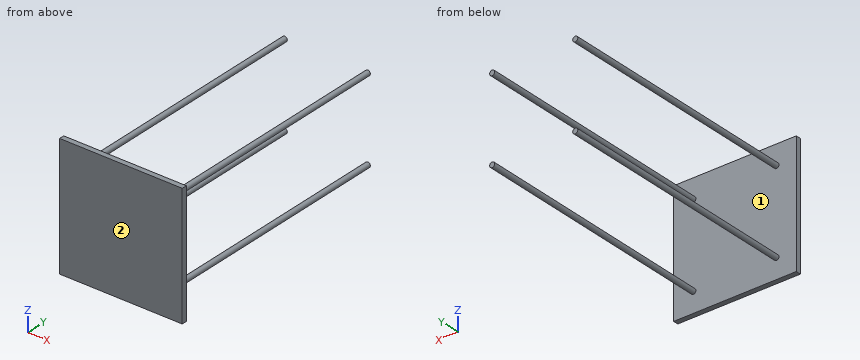
```python
from build123d import *

# Parameters (mm, degrees)
SKETCH1_W           = 120
SKETCH1_H           = 120
SKETCH1_R           = 2.5
BOSS_EXTRUDE1_DEPTH = 5
SKETCH1_3_R         = 2.5
BOSS_EXTRUDE2_DEPTH = 250


with BuildPart() as part:
    # Sketch1 → Boss-Extrude1 (new body)
    with BuildSketch(Plane(origin=(0, 0, 0), x_dir=(1, 0, 0), z_dir=(0, 1, 0))):
        Rectangle(SKETCH1_W, SKETCH1_H)
        with Locations(Location((-40.658639918, -40.658639918, 0), (0, 0, 270))):
            Circle(SKETCH1_R, mode=Mode.SUBTRACT)
        with Locations(Location((40.658639918, 40.658639918, 0), (0, 0, 270))):
            Circle(SKETCH1_R, mode=Mode.SUBTRACT)
        with Locations(Location((40.658639918, -40.658639918, 0), (0, 0, 270))):
            Circle(SKETCH1_R, mode=Mode.SUBTRACT)
        with Locations(Location((-40.658639918, 40.658639918, 0), (0, 0, 270))):
            Circle(SKETCH1_R, mode=Mode.SUBTRACT)
    extrude(amount=BOSS_EXTRUDE1_DEPTH)

    # Sketch1_3 → Boss-Extrude2 (add)
    with BuildSketch(Plane(origin=(0, 0, 0), x_dir=(1, 0, 0), z_dir=(0, 1, 0))):
        with Locations(Location((-40.658639918, -40.658639918, 0), (0, 0, 270))):
            Circle(SKETCH1_3_R)
        with Locations(Location((-40.658639918, 40.658639918, 0), (0, 0, 270))):
            Circle(SKETCH1_3_R)
        with Locations(Location((40.658639918, 40.658639918, 0), (0, 0, 270))):
            Circle(SKETCH1_3_R)
        with Locations(Location((40.658639918, -40.658639918, 0), (0, 0, 270))):
            Circle(SKETCH1_3_R)
    extrude(amount=BOSS_EXTRUDE2_DEPTH)


solid = part.part
```
For this review, take the finished solid that the model builds, in its own axes (mm). Face numbers are marked on the shaded views. A direction names the side the tool comes from. Round coordinates to 2 decimals unless told otherwise and drop trailing zeros. Write each loop counter-clockwise with the first axis right and the second up, starting at its lowest first coordinate (ties: lowest second). Pieces come first, ordered by that corner, then holes.
1) Take a section at B-B on z = 28.5. Give the boundary of the cut face in (x, y), then the cut area to 3 significant figures.
Answer below:
outline: (-60, 0) - (60, 0) - (60, 5) - (-60, 5) - close
area: 600 mm2
2) Machinability: for the marked faces 1 and 2, which of the approach directions +Z, -Z, +X, -X, +Y, -Y give a long, thin tool a straight path to every point of the face, cutting with its end or side? Answer none if there is none.
Answer below:
face 1: +Y
face 2: +Z, -Z, +X, -X, -Y
3) Take a section at A-A on y = 83.5. Give the boundary of the cut face in (x, z).
Answer below:
outline: circle Ø5 at (-40.66, -40.66); circle Ø5 at (-40.66, 40.66); circle Ø5 at (40.66, -40.66); circle Ø5 at (40.66, 40.66)
4) For line 1 along Y through (x, z) = (-51, -34); line 2 along Z through (x, y) = (42.5, 154); line 3 along X through (y, z) = (193, -42), list the stretches that pass through material, from the lowest coordinate up.
Answer below:
line 1: y = 0 to 5
line 2: z = -42.35 to -38.97, 38.97 to 42.35
line 3: x = -42.77 to -38.55, 38.55 to 42.77
5) Insertion check: pin 1 Ø2 at (y, z) = (26, 41.5) entering from +X; pin 2 Ø5 at (x, z) = (27.5, 16) entering from +Y. Each pin has a flat end and moves straight along its axis. Give the tip position at first contact, or say it passes through.
Answer below:
pin 1: stops at x = 43.16
pin 2: stops at y = 5
6) Take a section at C-C on x = 0.5. Give the boundary of the cut face in (y, z).
Answer below:
outline: (0, -60) - (5, -60) - (5, 60) - (0, 60) - close
